from build123d import *

# Parameters (mm, degrees)
SKIZZE1_W                                           = 115.555555556
SKIZZE1_H                                           = 155.555555556
AUFSATZ_LINEAR_AUSTRAGEN1_DEPTH                     = 704
SCHNITT_LINEAR_AUSTRAGEN1_DEPTH                     = 718.647872662
SCHNITT_LINEAR_AUSTRAGEN2_DEPTH                     = 724.292335414
SPIEGELN2_COPY_1_DEPTH                              = 718.647872662
SPIEGELN2_COPY_2_DEPTH                              = 718.647872662
STIRNSENKUNG_F_R_M8_SENKSCHRAUBE_KOPF_B_D           = 9
STIRNSENKUNG_F_R_M8_SENKSCHRAUBE_KOPF_B_CBORE_D     = 22
STIRNSENKUNG_F_R_M8_SENKSCHRAUBE_KOPF_B_CBORE_DEPTH = 8
STIRNSENKUNG_F_R_M8_SENKSCHRAUBE_KO_2_D             = 9
STIRNSENKUNG_F_R_M8_SENKSCHRAUBE_KO_2_CBORE_D       = 15
STIRNSENKUNG_F_R_M8_SENKSCHRAUBE_KO_2_CBORE_DEPTH   = 8


with BuildPart() as part:
    # Skizze1 → Aufsatz-Linear austragen1 (new body)
    with BuildSketch(Plane.XY):
        Rectangle(SKIZZE1_W, SKIZZE1_H)
    extrude(amount=AUFSATZ_LINEAR_AUSTRAGEN1_DEPTH)

    # Skizze2 → Schnitt-Linear austragen1 (cut, through all)
    with BuildSketch(Plane(origin=(57.777777778, 0, 0), x_dir=(0, 0, -1), z_dir=(1, 0, 0))):
        with BuildLine():
            Line((-704, 53.777777778), (-704, 77.777777778))
            Line((-704, 77.777777778), (-680, 77.777777778))
            ThreePointArc((-680, 77.777777778), (-696.970562748, 70.748340526), (-704, 53.777777778))
        make_face()
    schnitt_linear_austragen1 = extrude(amount=-SCHNITT_LINEAR_AUSTRAGEN1_DEPTH, mode=Mode.SUBTRACT)

    # Skizze3 → Schnitt-Linear austragen2 (cut, through all)
    with BuildSketch(Plane(origin=(0, 77.777777778, 0), x_dir=(1, 0, 0), z_dir=(0, 1, 0))):
        with BuildLine():
            Line((-57.777777778, -680), (-57.777777778, -704))
            Line((-57.777777778, -704), (-33.777777778, -704))
            ThreePointArc((-33.777777778, -704), (-50.748340526, -696.970562748), (-57.777777778, -680))
        make_face()
    schnitt_linear_austragen2 = extrude(amount=-SCHNITT_LINEAR_AUSTRAGEN2_DEPTH, mode=Mode.SUBTRACT)

    # Spiegeln1: Schnitt-Linear austragen1 across plane
    add(schnitt_linear_austragen1.mirror(Plane.ZX), mode=Mode.SUBTRACT)

    # Spiegeln2: Schnitt-Linear austragen2 across plane
    add(schnitt_linear_austragen2.mirror(Plane(origin=(0, 0, 0), x_dir=(0, 0, 1), z_dir=(1, 0, 0))), mode=Mode.SUBTRACT)

    # Spiegeln2 copy 1 sketch → Spiegeln2 copy 1 (cut, through all)
    with BuildSketch(Plane(origin=(-57.777777778, 0, 0), x_dir=(0, 0, -1), z_dir=(-1, 0, 0))):
        with BuildLine():
            Line((-704, 53.777777778), (-704, 77.777777778))
            Line((-704, 77.777777778), (-680, 77.777777778))
            ThreePointArc((-680, 77.777777778), (-696.970562748, 70.748340526), (-704, 53.777777778))
        make_face()
    extrude(amount=-SPIEGELN2_COPY_1_DEPTH, mode=Mode.SUBTRACT)

    # Spiegeln2 copy 2 sketch → Spiegeln2 copy 2 (cut, through all)
    with BuildSketch(Plane(origin=(-57.777777778, 0, 0), x_dir=(0, 0, -1), z_dir=(-1, 0, 0))):
        with BuildLine():
            Line((-704, -53.777777778), (-704, -77.777777778))
            Line((-704, -77.777777778), (-680, -77.777777778))
            ThreePointArc((-680, -77.777777778), (-696.970562748, -70.748340526), (-704, -53.777777778))
        make_face()
    extrude(amount=-SPIEGELN2_COPY_2_DEPTH, mode=Mode.SUBTRACT)

    # Stirnsenkung f_r M8 Senkschraube _Kopf B (through all)
    with Locations(Plane(origin=(0, 77.777777778, 0), x_dir=(1, 0, 0), z_dir=(0, 1, 0))):
        with Locations((0, -654), (0, -44)):
            CounterBoreHole(STIRNSENKUNG_F_R_M8_SENKSCHRAUBE_KOPF_B_D / 2, STIRNSENKUNG_F_R_M8_SENKSCHRAUBE_KOPF_B_CBORE_D / 2, STIRNSENKUNG_F_R_M8_SENKSCHRAUBE_KOPF_B_CBORE_DEPTH)

    # Stirnsenkung f_r M8 Senkschraube _Ko 2 (through all)
    with Locations(Plane(origin=(0, -77.777777778, 0), x_dir=(-1, 0, 0), z_dir=(0, -1, 0))):
        with Locations((0, -654), (0, -44)):
            CounterBoreHole(STIRNSENKUNG_F_R_M8_SENKSCHRAUBE_KO_2_D / 2, STIRNSENKUNG_F_R_M8_SENKSCHRAUBE_KO_2_CBORE_D / 2, STIRNSENKUNG_F_R_M8_SENKSCHRAUBE_KO_2_CBORE_DEPTH)


solid = part.part
Read the model definition and answer for the solid it produces. Units are mm, in the model's axes. A direction names the side the tool comes from. Round coordinates to 2 decimals unless told otherwise and drop trailing zeros.
Q1. This flat-tipped pin is pushed along its axis until it touches: pin 1 (13.5 mm diameter, centred on x = 0, z = 654, fed in from +Y). Where does it stop, or does it pass through?
Q2. Determine the mould class of faces 1 (the face through (-57.778, -1, 335)), 2 (the face through (-1, -77.778, 335)), 3 (the face through (5, 69.778, 44)) for opening direction X: released by +X, released by -X, zero draft, split by the parting line, or undercut.
Q3. Consider probe 1 along Z at (x, y) = (0, 41); probe 2 along X at (y, z) = (-75.25, 654); probe 3 along Z at (x, y) = (0, -71). Determine where each line is inside the solid, lowest interval first.
Q4. Which of the six approach directions +Z, -Z, +X, -X, +Y, -Y give full straight-line access (tool end or side, diameter ignored) to faces 4 (the face through (-2.38, 73.83, 664.74)), 5 (the face through (0.809, 70.934, 696.783)), 6 (the face through (0.976, -73.834, 646.564))?
Output:
1. pin 1: stops at y = 69.78
2. face 1: released by -X
2. face 2: zero draft
2. face 3: undercut
3. probe 1: z = 0 to 39.5, 48.5 to 649.5, 658.5 to 704
3. probe 2: x = -57.78 to -7.5, 7.5 to 57.78
3. probe 3: z = 0 to 36.5, 51.5 to 646.5, 661.5 to 696.72
4. face 4: +Y
4. face 5: +Z, +X, -X, +Y
4. face 6: -Y
